Design review of the part built by this model. Coordinates are the model's own, in mm. Give positions to 0.01 mm unless a question says otherwise; leave off trailing zeros. Write each loop counter-clockwise with the first axis right and the second up, starting at its lowest first coordinate (ties: lowest second). Pieces come first, ordered by that corner, then holes. Notation, with made-up numbers: M 73.5,11 L 81.5,11 A7 cw 81.5,18 Z; hole C 29.25,84 d3. An arc over 180 degrees is marked long. Answer in a Markdown table with one row per item.
```python
from build123d import *

# Parameters (mm, degrees)
BOSS_EXTRU_1_DEPTH      = 4.3
ESQUISSE2_W             = 5.6
ESQUISSE2_H             = 2.4
BOSS_EXTRU_2_DEPTH      = 0.65
ESQUISSE3_W             = 2.4
ESQUISSE3_H             = 4.95
BOSS_EXTRU_3_DEPTH      = 2.4
ESQUISSE4_W             = 8
ESQUISSE4_H             = 2.4
BOSS_EXTRU_4_DEPTH      = 3.85
ESQUISSE5_W             = 2.4
ESQUISSE5_H             = 8.8
BOSS_EXTRU_5_DEPTH      = 3.2
ESQUISSE6_W             = 2.35
ESQUISSE6_H             = 0.9
BOSS_EXTRU_6_DEPTH      = 3.1
ESQUISSE7_W             = 0.9
ESQUISSE7_H             = 4.3
BOSS_EXTRU_7_DEPTH      = 0.4
ESQUISSE8_W             = 0.9
ESQUISSE8_H             = 4.3
BOSS_EXTRU_8_DEPTH      = 0.4
ESQUISSE9_W             = 5.5
ESQUISSE9_H             = 8.8
BOSS_EXTRU_9_DEPTH      = 0.8
BOSS_EXTRU_10_DEPTH     = 2.4
ESQUISSE11_W            = 12
ESQUISSE11_H            = 5.5
BOSS_EXTRU_11_DEPTH     = 0.8
ENL_V_MAT_EXTRU_1_DEPTH = 1.6
ENL_V_MAT_EXTRU_2_REACH = 12.401
ESQUISSE13_W            = 1.425
ESQUISSE13_H            = 1.6
ENL_V_MAT_EXTRU_3_REACH = 12.401
ESQUISSE14_W            = 1.425
ESQUISSE14_H            = 1.6
ENL_V_MAT_EXTRU_4_DEPTH = 1.6
CONG_1_R                = 0.25


with BuildPart() as part:
    # Esquisse1 → Boss.-Extru.1 (new body)
    with BuildSketch(Plane.XZ.offset(2.15)):
        with BuildLine():
            Line((1.9, 0.4), (2.8, 0.4))
            Line((2.8, 0.4), (2.8, 5.5))
            Line((2.8, 5.5), (-2.8, 5.5))
            Line((-2.8, 5.5), (-2.8, 0.4))
            Line((-2.8, 0.4), (-1.9, 0.4))
            ThreePointArc((-1.9, 0.4), (-1.72, 0.7), (-1.9, 1))
            Line((-1.9, 1), (-1.9, 3.1))
            Line((-1.9, 3.1), (1.9, 3.1))
            Line((1.9, 3.1), (1.9, 1))
            ThreePointArc((1.9, 1), (1.72, 0.7), (1.9, 0.4))
        make_face()
    extrude(amount=-BOSS_EXTRU_1_DEPTH)

    # Esquisse2 → Boss.-Extru.2 (add)
    with BuildSketch(Plane.XZ.offset(2.15)):
        with Locations((0, 4.3)):
            Rectangle(ESQUISSE2_W, ESQUISSE2_H)
    extrude(amount=BOSS_EXTRU_2_DEPTH)

    # Esquisse3 → Boss.-Extru.3 (add)
    with BuildSketch(Plane.ZY.offset(2.8)):
        with Locations((4.3, -0.325)):
            Rectangle(ESQUISSE3_W, ESQUISSE3_H)
    extrude(amount=BOSS_EXTRU_3_DEPTH)

    # Esquisse4 → Boss.-Extru.4 (add)
    with BuildSketch(Plane(origin=(0, 2.15, 0), x_dir=(-1, 0, 0), z_dir=(0, 1, 0))):
        with Locations((1.2, 4.3)):
            Rectangle(ESQUISSE4_W, ESQUISSE4_H)
    extrude(amount=BOSS_EXTRU_4_DEPTH)

    # Esquisse5 → Boss.-Extru.5 (add)
    with BuildSketch(Plane(origin=(2.8, 0, 0), x_dir=(0, 0, -1), z_dir=(1, 0, 0))):
        with Locations((-4.3, 1.6)):
            Rectangle(ESQUISSE5_W, ESQUISSE5_H)
    extrude(amount=BOSS_EXTRU_5_DEPTH)

    # Esquisse6 → Boss.-Extru.6 (add)
    with BuildSketch(Plane(origin=(0, 0, 3.1), x_dir=(-1, 0, 0), z_dir=(0, 0, -1))):
        Polygon((5.2, 5.2), (0.475, 5.2), (0.475, 2.8), (1.175, 2.8), (1.175, 1.9), (-1.175, 1.9), (-1.175, 2.8), (-0.475, 2.8), (-0.475, 5.2), (-5.2, 5.2), (-5.2, -2.8), (-6, -2.8), (-6, 6), (5.2, 6), align=None)
        with Locations((0, -2.35)):
            Rectangle(ESQUISSE6_W, ESQUISSE6_H)
    extrude(amount=BOSS_EXTRU_6_DEPTH)

    # Esquisse7 → Boss.-Extru.7 (add)
    with BuildSketch(Plane(origin=(0, 0, 0.4), x_dir=(-1, 0, 0), z_dir=(0, 0, -1))):
        with Locations((2.35, 0)):
            Rectangle(ESQUISSE7_W, ESQUISSE7_H)
    extrude(amount=BOSS_EXTRU_7_DEPTH)

    # Esquisse8 → Boss.-Extru.8 (add)
    with BuildSketch(Plane(origin=(0, 0, 0.4), x_dir=(-1, 0, 0), z_dir=(0, 0, -1))):
        with Locations((-2.35, 0)):
            Rectangle(ESQUISSE8_W, ESQUISSE8_H)
    extrude(amount=BOSS_EXTRU_8_DEPTH)

    # Esquisse9 → Boss.-Extru.9 (add)
    with BuildSketch(Plane.ZY.offset(5.2)):
        with Locations((2.75, 1.6)):
            Rectangle(ESQUISSE9_W, ESQUISSE9_H)
    extrude(amount=BOSS_EXTRU_9_DEPTH)

    # Esquisse10 → Boss.-Extru.10 (add)
    with BuildSketch(Plane.XZ.offset(2.8)):
        Polygon((-0.475, 3.1), (-5.2, 3.1), (-5.2, 0), (-6, 0), (-6, 5.5), (6, 5.5), (6, 0), (5.2, 0), (5.2, 3.1), (0.475, 3.1), (0.475, 0), (-0.475, 0), align=None)
    extrude(amount=BOSS_EXTRU_10_DEPTH)

    # Esquisse11 → Boss.-Extru.11 (add)
    with BuildSketch(Plane.XZ.offset(5.2)):
        with Locations((0, 2.75)):
            Rectangle(ESQUISSE11_W, ESQUISSE11_H)
    extrude(amount=BOSS_EXTRU_11_DEPTH)

    # Esquisse12 → Enlèv. mat.-Extru.1 (cut)
    with BuildSketch(Plane(origin=(0, 0, 3.1), x_dir=(-1, 0, 0), z_dir=(0, 0, -1))):
        Polygon((-1.9, 0.475), (-1.175, 0.475), (-1.175, 2.8), (-0.475, 2.8), (-0.475, 5.2), (-5.2, 5.2), (-5.2, -5.2), (-0.475, -5.2), (-0.475, -2.8), (-1.175, -2.8), (-1.175, -0.475), (-1.9, -0.475), (-1.9, -2.15), (-2.8, -2.15), (-2.8, 2.15), (-1.9, 2.15), align=None)
    extrude(amount=-ENL_V_MAT_EXTRU_1_DEPTH, mode=Mode.SUBTRACT)

    # Esquisse13 → Enlèv. mat.-Extru.2 (cut, up to next)
    with BuildSketch(Plane(origin=(0.475, 0, 0), x_dir=(0, -1, 0), z_dir=(-1, 0, 0)), mode=Mode.PRIVATE) as enl_v_mat_extru_2_sk1:
        with Locations((-1.1875, 3.9)):
            Rectangle(ESQUISSE13_W, ESQUISSE13_H)
    enl_v_mat_extru_2_tool1 = extrude(enl_v_mat_extru_2_sk1.sketch, amount=-ENL_V_MAT_EXTRU_2_REACH, mode=Mode.PRIVATE) & part.part
    add(enl_v_mat_extru_2_tool1.solids().sort_by_distance((0.475, 1.1875, 3.9))[0], mode=Mode.SUBTRACT)

    # Esquisse14 → Enlèv. mat.-Extru.3 (cut, up to next)
    with BuildSketch(Plane(origin=(0.475, 0, 0), x_dir=(0, -1, 0), z_dir=(-1, 0, 0)), mode=Mode.PRIVATE) as enl_v_mat_extru_3_sk1:
        with Locations((1.1875, 3.9)):
            Rectangle(ESQUISSE14_W, ESQUISSE14_H)
    enl_v_mat_extru_3_tool1 = extrude(enl_v_mat_extru_3_sk1.sketch, amount=-ENL_V_MAT_EXTRU_3_REACH, mode=Mode.PRIVATE) & part.part
    add(enl_v_mat_extru_3_tool1.solids().sort_by_distance((0.475, -1.1875, 3.9))[0], mode=Mode.SUBTRACT)

    # Esquisse15 → Enlèv. mat.-Extru.4 (cut)
    with BuildSketch(Plane(origin=(0, 0, 3.1), x_dir=(-1, 0, 0), z_dir=(0, 0, -1))):
        Polygon((0.475, 0.475), (1.9, 0.475), (1.9, 2.15), (2.8, 2.15), (2.8, -2.15), (1.9, -2.15), (1.9, -0.475), (0.475, -0.475), (0.475, -1.9), (1.175, -1.9), (1.175, -2.8), (0.475, -2.8), (0.475, -5.2), (5.2, -5.2), (5.2, 5.2), (0.475, 5.2), (0.475, 2.8), (1.175, 2.8), (1.175, 1.9), (0.475, 1.9), align=None)
    extrude(amount=-ENL_V_MAT_EXTRU_4_DEPTH, mode=Mode.SUBTRACT)

    # Congé1
    cong_1_edges = [part.edges().sort_by_distance(p)[0] for p in [
        (-6, 0, 5.5),
        (-6, 6, 2.75),
        (6, -6, 2.75),
        (0, -6, 5.5),
        (-6, -6, 2.75),
        (0, 6, 5.5),
        (6, 6, 2.75),
        (6, 0, 5.5),
    ]]
    fillet(cong_1_edges, radius=CONG_1_R)


solid = part.part
```
1) To check wall thickness, follow probe 1 along Y at (x, z) = (1, 3.8) (3 decimals); probe 2 along Y at (x, z) = (2.25, 2.8); probe 3 along X at (y, z) = (5, 3.7) (3 decimals). State the ranges of each line that lie inside material, in increasing order. Write a range as [from, to].
Geometry says:
| item | result |
|---|---|
| probe 1 | [-6, -5.2], [-2.8, -1.9], [-0.475, 0.475], [1.9, 2.8], [5.2, 6] |
| probe 2 | [-6, -5.2], [-2.15, 2.15], [5.2, 6] |
| probe 3 | [-6, -5.2], [-0.475, 0.475], [5.2, 6] |
2) The part is to be moulded in two halves that separate along Y. For faces 1 (the face through (-3, -5.2, 2)), 2 (the face through (0, 6, 3)), 3 (the face through (-6, 0, 3)), say which applies: released by +Y, released by -Y, zero draft, split by the parting line, or undercut.
Geometry says:
| item | result |
|---|---|
| face 1 | undercut |
| face 2 | released by +Y |
| face 3 | zero draft |
3) Add section B-B (y = -3). Write out the cut boundary in (x, z) (3 decimals), and give its area (3 significant figures).
Geometry says:
| item | result |
|---|---|
| outline | M -6,0 L -5.2,0 L -5.2,4.7 L -0.475,4.7 L -0.475,0 L 0.475,0 L 0.475,4.7 L 5.2,4.7 L 5.2,0 L 6,0 L 6,5.25 A0.25 ccw 5.75,5.5 L -5.75,5.5 A0.25 ccw -6,5.25 Z |
| area | 21.6 mm^2 |
4) Add section C-C (x = -2.25). Write out the cut boundary in (y, z).
Geometry says:
| item | result |
|---|---|
| outline | M -6,0 L -5.2,0 L -5.2,4.7 L -2.15,4.7 L -2.15,0 L 2.15,0 L 2.15,4.7 L 5.2,4.7 L 5.2,0 L 6,0 L 6,5.25 A0.25 ccw 5.75,5.5 L -5.75,5.5 A0.25 ccw -6,5.25 Z |
5) Insertion check: P1, Ø1.4, axis at x = -3.5, y = -2.5, coming from the -Z side. The pin has a flat end and moves straight along its axis. Give the tip position at first contact, or say it passes through.
Geometry says:
| item | result |
|---|---|
| P1 | z = 4.7 |
6) Add section A-A (z = 2). Count the separate pieces of the cut face and the enclosed holes in it, and give its area (3 significant figures).
Geometry says:
| item | result |
|---|---|
| separate pieces | 3 |
| enclosed holes | 1 |
| area | 52.3 mm^2 |
